from build123d import *

# Parameters (mm, degrees)
BOSS_EXTRUDE3_DEPTH     = 5
SKETCH2_W               = 30
SKETCH2_H               = 30
SKETCH2_W_2             = 20
SKETCH2_H_2             = 20
BOSS_EXTRUDE4_DEPTH     = 10
SKETCH3_R               = 1.5
CUT_EXTRUDE1_DEPTH      = 5
CUT_EXTRUDE2_DEPTH      = 37.742346142
CUT_EXTRUDE2_DEPTH_BACK = 37.742346142
SKETCH4_W               = 20
SKETCH4_H               = 8
CUT_EXTRUDE3_DEPTH      = 37.742346142
CUT_EXTRUDE3_DEPTH_BACK = 37.742346142
SKETCH5_W               = 20
SKETCH5_H               = 7


with BuildPart() as part:
    # Sketch1 → Boss-Extrude3 (new body)
    with BuildSketch(Plane(origin=(0, 0, 0), x_dir=(1, 0, 0), z_dir=(0, 1, 0))):
        Polygon((-15, 15), (-15, -15), (15, -15), (15, -10.5), (12.5, -10.5), (-12.5, -10.5), (-12.5, 10.5), (12.5, 10.5), (15, 10.5), (15, 15), align=None)
    extrude(amount=BOSS_EXTRUDE3_DEPTH)

    # Sketch2 → Boss-Extrude4 (add)
    with BuildSketch(Plane(origin=(0, 5, 0), x_dir=(1, 0, 0), z_dir=(0, 1, 0))):
        Rectangle(SKETCH2_W, SKETCH2_H)
        Rectangle(SKETCH2_W_2, SKETCH2_H_2, mode=Mode.SUBTRACT)
    extrude(amount=BOSS_EXTRUDE4_DEPTH)

    # Sketch3 → Cut-Extrude1 (cut)
    with BuildSketch(Plane(origin=(0, 15, 0), x_dir=(1, 0, 0), z_dir=(0, 1, 0))):
        with Locations(Location((-12, 12, 0), (0, 0, 270))):
            Circle(SKETCH3_R)
        with Locations(Location((12, 12, 0), (0, 0, 270))):
            Circle(SKETCH3_R)
        with Locations(Location((12, -12, 0), (0, 0, 270))):
            Circle(SKETCH3_R)
        with Locations(Location((-12, -12, 0), (0, 0, 270))):
            Circle(SKETCH3_R)
    extrude(amount=-CUT_EXTRUDE1_DEPTH, mode=Mode.SUBTRACT)

    # Sketch4 → Cut-Extrude2 (cut, two sides: drawn at the far end of the back side and taken through both)
    with BuildSketch(Plane(origin=(0, 0, -15), x_dir=(-1, 0, 0), z_dir=(0, 0, -1)).offset(-CUT_EXTRUDE2_DEPTH_BACK)):
        with Locations((0, 9)):
            Rectangle(SKETCH4_W, SKETCH4_H)
    extrude(amount=CUT_EXTRUDE2_DEPTH + CUT_EXTRUDE2_DEPTH_BACK, mode=Mode.SUBTRACT)

    # Sketch5 → Cut-Extrude3 (cut, two sides: drawn at the far end of the back side and taken through both)
    with BuildSketch(Plane.ZY.offset(15).offset(-CUT_EXTRUDE3_DEPTH_BACK)):
        with Locations((0, 9.5)):
            Rectangle(SKETCH5_W, SKETCH5_H)
    extrude(amount=CUT_EXTRUDE3_DEPTH + CUT_EXTRUDE3_DEPTH_BACK, mode=Mode.SUBTRACT)


solid = part.part
Verification items for the finished model (mm, model axes). A direction names the side the tool comes from. Give positions to 0.01 mm unless a question says otherwise; leave off trailing zeros. Write each loop counter-clockwise with the first axis right and the second up, starting at its lowest first coordinate (ties: lowest second). Pieces come first, ordered by that corner, then holes. Notation, with made-up numbers: (40, 80) - (49, 80) arc R12 ccw to (49, 103) - close; hole circle Ø3 at (24, 52). An arc over 180 degrees is marked (long way). Answer as CSV lines item,"result". Start each with the question number.
1. Sectioned sample at B-B (z = -12). Record the boundary of the cut face in (x, y).
2. Draft check along X on faces 5 (the face through (-12, 9, 10)), 6 (the face through (-12.5, 2, 0)), 7 (the face through (0, 14, 10)). Enter one of: pulls with the +X half, pulls with the -X half, needs draft (parallel to the pull), parting line crosses it, or undercut.
3. Sectioned sample at D-D (y = 2.75). Record the boundary of the cut face in (x, z), then the cut area to 4 significant figures.
4. Sectioned sample at C-C (x = -7.25). Record the boundary of the cut face in (y, z), then the cut area to 3 significant figures.
5. Sectioned sample at A-A (x = -12). Record the boundary of the cut face in (y, z), then the cut area to 3 significant figures.
6. Thickness scan on line 1 (X direction, y = 13.3, z = 12); line 2 (X direction, y = 12.15, z = -12); line 3 (Y direction, x = 13, z = 6.25). Record the ranges inside material, lowest first.
7. Set-up check for faces 1 (the face through (0, 13, -12)), 2 (the face through (12, 5, 0)), 3 (the face through (-12, 13, 0)), 4 (the face through (12.07, 12.54, -13.5)): record each of +Z, -Z, +X, -X, +Y, -Y from which the full face is reachable in a straight line by a thin tool's end or side.
8. Depth check by flat-ended pin: pin 1 (1.5 mm diameter, centred on y = 2, z = 1.5, fed in from +X); pin 2 (4 mm diameter, centred on y = 9, z = -6, fed in from +X); pin 3 (2 mm diameter, centred on y = 6.5, z = -8, fed in from -X); pin 4 (1.2 mm diameter, centred on x = -11, z = -4.5, fed in from -Y). Enter the tip coordinate at first touch or a pass-through.
Derived:
1,outline,"(-15, 0) - (15, 0) - (15, 15) - (13.5, 15) - (13.5, 10) - (10.5, 10) - (10.5, 15) - (-10.5, 15) - (-10.5, 10) - (-13.5, 10) - (-13.5, 15) - (-15, 15) - close; hole (-10, 5) - (10, 5) - (10, 13) - (-10, 13) - close"
2,face 5,"needs draft"
2,face 6,"pulls with the +X half"
2,face 7,"undercut"
3,outline,"(-15, -15) - (15, -15) - (15, -10.5) - (-12.5, -10.5) - (-12.5, 10.5) - (15, 10.5) - (15, 15) - (-15, 15) - close"
3,area,"322.5 mm²"
4,outline,"(0, -15) - (5, -15) - (5, -10.5) - (0, -10.5) - close; (0, 10.5) - (5, 10.5) - (5, 15) - (0, 15) - close; (13, -15) - (15, -15) - (15, -10) - (13, -10) - close; (13, 10) - (15, 10) - (15, 15) - (13, 15) - close"
4,area,"65.0 mm²"
5,outline,"(0, -15) - (15, -15) - (15, -13.5) - (10, -13.5) - (10, -10.5) - (15, -10.5) - (15, 10.5) - (10, 10.5) - (10, 13.5) - (15, 13.5) - (15, 15) - (0, 15) - (0, 10.5) - (5, 10.5) - (5, -10.5) - (0, -10.5) - close; hole (6, -10) - (13, -10) - (13, 10) - (6, 10) - close"
5,area,"175 mm²"
6,line 1,"-15 to -13.5, -10.5 to 10.5, 13.5 to 15"
6,line 2,"-15 to -13.5, -10.5 to -10, 10 to 10.5, 13.5 to 15"
6,line 3,"5 to 6, 13 to 15"
7,face 1,"+Z, -Z"
7,face 2,"+X, -Y"
7,face 3,"+X, -X"
7,face 4,"+Y"
8,pin 1,"x = -12.5"
8,pin 2,"through"
8,pin 3,"x = -15"
8,pin 4,"y = 5"
